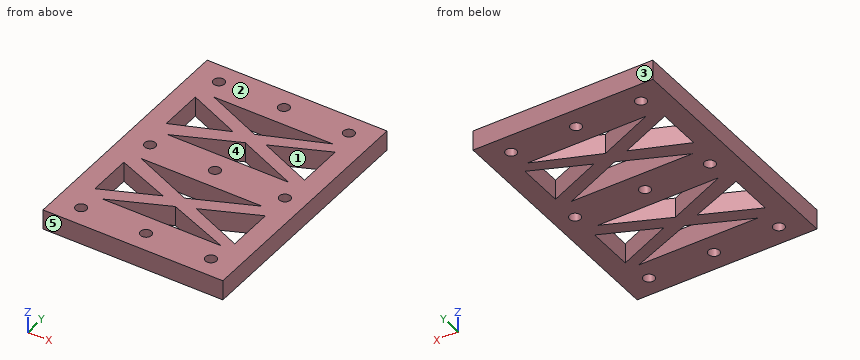
from build123d import *

# Parameters (mm, degrees)
SKETCH_1_W          = 72
SKETCH_1_H          = 100
EXTRUDE_1_DEPTH     = 8
CUT_EXTRUDE_1_REACH = 64.129
SKETCH_2_R          = 2.2
SKETCH_2_W          = 56
SKETCH_2_H          = 26
EXTRUDE_2_DEPTH     = 8


with BuildPart() as part:
    # 草图1 → 凸台-拉伸1 (new body)
    with BuildSketch(Plane.XY):
        Rectangle(SKETCH_1_W, SKETCH_1_H)
    extrude(amount=EXTRUDE_1_DEPTH)

    # 草图2 → 切除-拉伸1 (cut, up to next)
    with BuildSketch(Plane.XY.offset(8), mode=Mode.PRIVATE) as cut_extrude_1_sk1:
        with Locations((-26, -42)):
            Circle(SKETCH_2_R)
    cut_extrude_1_tool1 = extrude(cut_extrude_1_sk1.sketch, amount=-CUT_EXTRUDE_1_REACH, mode=Mode.PRIVATE) & part.part
    # 草图2 → 切除-拉伸1 (cut, up to next)
    with BuildSketch(Plane.XY.offset(8), mode=Mode.PRIVATE) as cut_extrude_1_sk2:
        with Locations((0, -42)):
            Circle(SKETCH_2_R)
    cut_extrude_1_tool2 = extrude(cut_extrude_1_sk2.sketch, amount=-CUT_EXTRUDE_1_REACH, mode=Mode.PRIVATE) & part.part
    # 草图2 → 切除-拉伸1 (cut, up to next)
    with BuildSketch(Plane.XY.offset(8), mode=Mode.PRIVATE) as cut_extrude_1_sk3:
        with Locations((26, -42)):
            Circle(SKETCH_2_R)
    cut_extrude_1_tool3 = extrude(cut_extrude_1_sk3.sketch, amount=-CUT_EXTRUDE_1_REACH, mode=Mode.PRIVATE) & part.part
    # 草图2 → 切除-拉伸1 (cut, up to next)
    with BuildSketch(Plane.XY.offset(8), mode=Mode.PRIVATE) as cut_extrude_1_sk4:
        with Locations((26, 42)):
            Circle(SKETCH_2_R)
    cut_extrude_1_tool4 = extrude(cut_extrude_1_sk4.sketch, amount=-CUT_EXTRUDE_1_REACH, mode=Mode.PRIVATE) & part.part
    # 草图2 → 切除-拉伸1 (cut, up to next)
    with BuildSketch(Plane.XY.offset(8), mode=Mode.PRIVATE) as cut_extrude_1_sk5:
        with Locations((0, 42)):
            Circle(SKETCH_2_R)
    cut_extrude_1_tool5 = extrude(cut_extrude_1_sk5.sketch, amount=-CUT_EXTRUDE_1_REACH, mode=Mode.PRIVATE) & part.part
    # 草图2 → 切除-拉伸1 (cut, up to next)
    with BuildSketch(Plane.XY.offset(8), mode=Mode.PRIVATE) as cut_extrude_1_sk6:
        with Locations((-26, 42)):
            Circle(SKETCH_2_R)
    cut_extrude_1_tool6 = extrude(cut_extrude_1_sk6.sketch, amount=-CUT_EXTRUDE_1_REACH, mode=Mode.PRIVATE) & part.part
    # 草图2 → 切除-拉伸1 (cut, up to next)
    with BuildSketch(Plane.XY.offset(8), mode=Mode.PRIVATE) as cut_extrude_1_sk7:
        with Locations((-26, 0)):
            Circle(SKETCH_2_R)
    cut_extrude_1_tool7 = extrude(cut_extrude_1_sk7.sketch, amount=-CUT_EXTRUDE_1_REACH, mode=Mode.PRIVATE) & part.part
    # 草图2 → 切除-拉伸1 (cut, up to next)
    with BuildSketch(Plane.XY.offset(8), mode=Mode.PRIVATE) as cut_extrude_1_sk8:
        Circle(SKETCH_2_R)
    cut_extrude_1_tool8 = extrude(cut_extrude_1_sk8.sketch, amount=-CUT_EXTRUDE_1_REACH, mode=Mode.PRIVATE) & part.part
    # 草图2 → 切除-拉伸1 (cut, up to next)
    with BuildSketch(Plane.XY.offset(8), mode=Mode.PRIVATE) as cut_extrude_1_sk9:
        with Locations((28, 0)):
            Circle(SKETCH_2_R)
    cut_extrude_1_tool9 = extrude(cut_extrude_1_sk9.sketch, amount=-CUT_EXTRUDE_1_REACH, mode=Mode.PRIVATE) & part.part
    # 草图2 → 切除-拉伸1 (cut, up to next)
    with BuildSketch(Plane.XY.offset(8), mode=Mode.PRIVATE) as cut_extrude_1_sk10:
        with Locations((0, 21)):
            Rectangle(SKETCH_2_W, SKETCH_2_H)
    cut_extrude_1_tool10 = extrude(cut_extrude_1_sk10.sketch, amount=-CUT_EXTRUDE_1_REACH, mode=Mode.PRIVATE) & part.part
    # 草图2 → 切除-拉伸1 (cut, up to next)
    with BuildSketch(Plane.XY.offset(8), mode=Mode.PRIVATE) as cut_extrude_1_sk11:
        with Locations((0, -21)):
            Rectangle(SKETCH_2_W, SKETCH_2_H)
    cut_extrude_1_tool11 = extrude(cut_extrude_1_sk11.sketch, amount=-CUT_EXTRUDE_1_REACH, mode=Mode.PRIVATE) & part.part
    add(cut_extrude_1_tool1.solids().sort_by_distance((-26, -42, 8))[0], mode=Mode.SUBTRACT)
    add(cut_extrude_1_tool2.solids().sort_by_distance((0, -42, 8))[0], mode=Mode.SUBTRACT)
    add(cut_extrude_1_tool3.solids().sort_by_distance((26, -42, 8))[0], mode=Mode.SUBTRACT)
    add(cut_extrude_1_tool4.solids().sort_by_distance((26, 42, 8))[0], mode=Mode.SUBTRACT)
    add(cut_extrude_1_tool5.solids().sort_by_distance((0, 42, 8))[0], mode=Mode.SUBTRACT)
    add(cut_extrude_1_tool6.solids().sort_by_distance((-26, 42, 8))[0], mode=Mode.SUBTRACT)
    add(cut_extrude_1_tool7.solids().sort_by_distance((-26, 0, 8))[0], mode=Mode.SUBTRACT)
    add(cut_extrude_1_tool8.solids().sort_by_distance((0, 0, 8))[0], mode=Mode.SUBTRACT)
    add(cut_extrude_1_tool9.solids().sort_by_distance((28, 0, 8))[0], mode=Mode.SUBTRACT)
    add(cut_extrude_1_tool10.solids().sort_by_distance((0, 21, 8))[0], mode=Mode.SUBTRACT)
    add(cut_extrude_1_tool11.solids().sort_by_distance((0, -21, 8))[0], mode=Mode.SUBTRACT)

    # 草图3 → 凸台-拉伸2 (add)
    with BuildSketch(Plane.XY.offset(8)):
        Polygon((-28, 30.60122868), (-6.768682564, 21.407188314), (-28, 12.93157869), (-28, 8), (-24.288219299, 8), (-0.025829724, 18.487253581), (24.191837476, 8), (28, 8), (28, 11.903155093), (6.450556004, 21.286627452), (28, 30.60122868), (28, 34), (24.776184912, 34), (-0.016552798, 24.102660047), (-22.746110137, 34), (-28, 34), align=None)
        Polygon((-28, -8), (-24.288219299, -8), (-0.025829724, -18.487253581), (24.191837476, -8), (28, -8), (28, -11.903155093), (6.450556004, -21.286627452), (28, -30.60122868), (28, -34), (24.776184912, -34), (-0.016552798, -24.102660047), (-22.746110137, -34), (-28, -34), (-28, -30.60122868), (-6.768682564, -21.407188314), (-28, -12.93157869), align=None)
    extrude(amount=-EXTRUDE_2_DEPTH)


solid = part.part
Design review of the part built by this model. Coordinates are the model's own, in mm. Face numbers are marked on the shaded views. A direction names the side the tool comes from. Coordinates: 2 decimals unless noted, no trailing zeros. Order: outer loops, then holes, each group sorted by start corner. A loop starts at its lowest first (then second) coordinate and runs counter-clockwise, first axis right, second up. Notation, with made-up numbers: M 21.25,11 L 72.25,11 A12 ccw 72.25,21 Z; hole C -33.75,12 d3. An arc over 180 degrees is marked long. Use a Markdown table: item, result.
(1) Add section D-D (y = -33). Give the boundary of the cut face in (x, z), then the cut area to 3 significant figures.
Worked answers:
| item | result |
|---|---|
| outline | M -36,0 L -20.45,0 L -20.45,8 L -36,8 Z; M 22.27,0 L 36,0 L 36,8 L 22.27,8 Z |
| area | 234 mm2 |
(2) Add section C-C (x = 14.5). Give the boundary of the cut face in (y, z), then the cut area to 3 significant figures.
Worked answers:
| item | result |
|---|---|
| outline | M -50,0 L -34,0 L -34,8 L -50,8 Z; M -29.9,0 L -24.77,0 L -24.77,8 L -29.9,8 Z; M -17.78,0 L -12.2,0 L -12.2,8 L -17.78,8 Z; M -8,0 L 8,0 L 8,8 L -8,8 Z; M 12.2,0 L 17.78,0 L 17.78,8 L 12.2,8 Z; M 24.77,0 L 29.9,0 L 29.9,8 L 24.77,8 Z; M 34,0 L 50,0 L 50,8 L 34,8 Z |
| area | 555 mm2 |
(3) Add section B-B (x = -26). Give the boundary of the cut face in (y, z), then the cut area to 3 significant figures.
Worked answers:
| item | result |
|---|---|
| outline | M -50,0 L -44.2,0 L -44.2,8 L -50,8 Z; M -39.8,0 L -29.74,0 L -29.74,8 L -39.8,8 Z; M -13.73,0 L -2.2,0 L -2.2,8 L -13.73,8 Z; M 2.2,0 L 13.73,0 L 13.73,8 L 2.2,8 Z; M 29.74,0 L 39.8,0 L 39.8,8 L 29.74,8 Z; M 44.2,0 L 50,0 L 50,8 L 44.2,8 Z |
| area | 438 mm2 |
(4) For the marked faces 1 and 2, list the 3-axis set-ups (+Z, -Z, +X, -X, +Y, -Y) from which the entire face can be reached by the end or side of a thin tool; tool diameter is ignored.
Worked answers:
| item | result |
|---|---|
| face 1 | +Z, -Z |
| face 2 | +Z, +X, -X, +Y, -Y |
(5) For P1, Ø5, axis at x = -26, y = -42, coming from the +Z side, flat-tipped, find the tip position at first contact; note if it passes through.
Worked answers:
| item | result |
|---|---|
| P1 | stops at z = 8 |
(6) Add section A-A (y = 0). Give the boundary of the cut face in (x, z).
Worked answers:
| item | result |
|---|---|
| outline | M -36,0 L -28.2,0 L -28.2,8 L -36,8 Z; M -23.8,0 L -2.2,0 L -2.2,8 L -23.8,8 Z; M 2.2,0 L 25.8,0 L 25.8,8 L 2.2,8 Z; M 30.2,0 L 36,0 L 36,8 L 30.2,8 Z |
(7) Wall thickness on probe 1 along X at (y, z) = (-23.5, 2); probe 2 along X at (y, z) = (2, 2.75); probe 3 along Y at (x, z) = (-2.5, 6): over which ranges is each line inside the solid? List them lowest first.
Worked answers:
| item | result |
|---|---|
| probe 1 | x = -36 to -28, -11.6 to 11.57, 28 to 36 |
| probe 2 | x = -36 to -26.92, -25.08 to -0.92, 0.92 to 27.08, 28.92 to 36 |
| probe 3 | y = -50 to -34, -25.18 to -17.42, -8 to 8, 17.42 to 25.18, 34 to 50 |
(8) Draft analysis for pull direction Y (two halves, no side actions). For the marked faces 3, 4 and 5, state which applies: released by +Y, released by -Y, zero draft, split by the parting line, or undercut.
Worked answers:
| item | result |
|---|---|
| face 3 | released by +Y |
| face 4 | undercut |
| face 5 | released by -Y |
